from build123d import *

# Parameters (mm, degrees)
F0_W     = 63.5
F0_H     = 44.45
F1_DEPTH = 588.9625
F3_DEPTH = 25.4
F2_W     = 7.9375
F2_H     = 425.45
F4_DEPTH = 9.525
F6_DEPTH = 9.525
F5_W     = 9.525
F5_H     = 20.7645
F5_H_2   = 28.575
F7_DEPTH = 44.451
F8_SIZE  = 11.90625


with BuildPart() as f1:
    # F0 (on Top) → F1 (new body)
    with BuildSketch(Plane.XY):
        with Locations((31.75, 22.225)):
            Rectangle(F0_W, F0_H)
    extrude(amount=F1_DEPTH)

    # F2 (on face) → F3 (cut)
    with BuildSketch(Plane.YZ.offset(63.5)):
        Polygon((26.9875, 579.4375), (17.4625, 579.4375), (17.4625, 522.2875), (18.25625, 522.2875), (26.19375, 522.2875), (26.9875, 522.2875), align=None)
        Polygon((26.19375, 96.8375), (18.25625, 96.8375), (17.4625, 96.8375), (17.4625, 26.9875), (26.9875, 26.9875), (26.9875, 96.8375), align=None)
    extrude(amount=-F3_DEPTH, mode=Mode.SUBTRACT)

    # F2 (on face) → F4 (cut)
    with BuildSketch(Plane.YZ.offset(63.5)):
        with Locations((22.225, 309.5625)):
            Rectangle(F2_W, F2_H)
    extrude(amount=-F4_DEPTH, mode=Mode.SUBTRACT)

    # F5 (on face) → F6 (cut)
    with BuildSketch(Plane.XZ):
        Polygon((35.71875, 522.0335), (28.575, 522.0335), (27.78125, 522.0335), (27.78125, 96.8375), (35.71875, 96.8375), align=None)
    extrude(amount=-F6_DEPTH, mode=Mode.SUBTRACT)

    # F5 (on face) → F7 (cut, through all)
    with BuildSketch(Plane.XZ):
        with Locations((31.75, 569.05525)):
            Rectangle(F5_W, F5_H)
        Polygon((27.78125, 522.0335), (28.575, 522.0335), (35.71875, 522.0335), (36.5125, 522.0335), (36.5125, 542.798), (26.9875, 542.798), (26.9875, 522.0335), align=None)
        Polygon((35.71875, 96.8375), (27.78125, 96.8375), (26.9875, 96.8375), (26.9875, 68.2625), (36.5125, 68.2625), (36.5125, 96.8375), align=None)
        with Locations((31.75, 41.275)):
            Rectangle(F5_W, F5_H_2)
    extrude(amount=-F7_DEPTH, mode=Mode.SUBTRACT)

    # F8
    f8_edges = [f1.edges().sort_by_distance(p)[0] for p in [
        (63.5, 44.45, 294.48125),
        (0, 44.45, 294.48125),
        (63.5, 0, 294.48125),
        (0, 0, 294.48125),
    ]]
    chamfer(f8_edges, length=F8_SIZE)


solid = f1.part
Design review of the part built by this model. Coordinates are the model's own, in mm. A direction names the side the tool comes from. Round coordinates to 2 decimals unless told otherwise and drop trailing zeros. Write each loop counter-clockwise with the first axis right and the second up, starting at its lowest first coordinate (ties: lowest second). Pieces come first, ordered by that corner, then holes.
Item 1: Draft analysis for pull direction X (two halves, no side actions). For faces 6 (the flat face through (26.988, 22, 83)), 7 (the flat face through (27, 0, 290)), 8 (the flat face through (38.1, 22, 551)), state which applies: released by +X, released by -X, zero draft, split by the parting line, or undercut.
Item 2: For pin 1 Ø1.5 at (y, z) = (10, 438) entering from -X; pin 2 Ø10.5 at (x, z) = (59, 301) entering from -Y, all flat-tipped, find the tip position at first contact; note any pin that passes through.
Item 3: Consider section A-A on z = 440.5. Give the boundary of the cut face in (x, y) (3 decimals).
Item 4: Wall thickness on L1, parallel to Z at x = 50, y = 18; L2, parallel to X at y = 29, z = 86.5; L3, parallel to Z at x = 34, y = 33: over which ranges is each line inside the solid? List them lowest first.
Item 5: Consider section B-B on x = 5.5. Give the boundary of the cut face in (y, z).
Item 6: For faces 1 (the flat face through (48, 22, 522.288)), 2 (the flat face through (27.781, 5, 312)), 3 (the flat face through (31, 23, 588.962)), 4 (the flat face through (26.988, 22, 41)), 5 (the flat face through (63.5, 27, 290)), list the 3-axis set-ups (+Z, -Z, +X, -X, +Y, -Y) from which the entire face can be reached by the end or side of a thin tool; tool diameter is ignored.
Check values:
1. face 6: undercut
1. face 7: zero draft
1. face 8: released by +X
2. pin 1: stops at x = 1.16
2. pin 2: stops at y = 2.16
3. outline: (0, 11.906) - (11.906, 0) - (27.781, 0) - (27.781, 9.525) - (35.719, 9.525) - (35.719, 0) - (51.594, 0) - (63.5, 11.906) - (63.5, 18.256) - (53.975, 18.256) - (53.975, 26.194) - (63.5, 26.194) - (63.5, 32.544) - (51.594, 44.45) - (11.906, 44.45) - (0, 32.544) - close
4. L1: z = 0 to 26.99, 96.84 to 522.29, 579.44 to 588.96
4. L2: x = 0 to 26.99, 36.51 to 63.5
4. L3: z = 0 to 26.99, 55.56 to 68.26, 96.84 to 522.03, 542.8 to 558.67, 579.44 to 588.96
5. outline: (6.41, 0) - (38.04, 0) - (38.04, 588.96) - (6.41, 588.96) - close
6. face 1: +X
6. face 2: -Y
6. face 3: +Z, +X, -X, +Y, -Y
6. face 4: +Y, -Y
6. face 5: +Z, -Z, +X, +Y, -Y
